```python
from build123d import *

# Parameters (mm, degrees)
BOSS_EXTRUDE2_DEPTH = 331.382
SKETCH3_W           = 66
SKETCH3_H           = 122
CUT_EXTRUDE2_DEPTH  = 128.0000001
SKETCH4_W           = 180
SKETCH4_H           = 60.8
CUT_EXTRUDE3_DEPTH  = 332.3820001
SKETCH5_W           = 260
SKETCH5_H           = 20
CUT_EXTRUDE4_DEPTH  = 332.3820001


with BuildPart() as part:
    # Sketch2 → Boss-Extrude2 (new body)
    with BuildSketch(Plane.XY):
        with BuildLine():
            Line((-127, 127), (127, 127))
            add(Edge.make_bspline(
                [(-127, 127), (0, -127), (127, 127)],
                knots=[0.056028396, 0.056028396, 0.056028396, 0.943971604, 0.943971604, 0.943971604], degree=2))
        make_face()
    extrude(amount=BOSS_EXTRUDE2_DEPTH)

    # Sketch3 → Cut-Extrude2 (cut, through all)
    with BuildSketch(Plane(origin=(0, 127, 0), x_dir=(1, 0, 0), z_dir=(0, 1, 0))):
        with Locations((0, -82.8455)):
            Rectangle(SKETCH3_W, SKETCH3_H)
        with Locations((0, -248.5365)):
            Rectangle(SKETCH3_W, SKETCH3_H)
    extrude(amount=-CUT_EXTRUDE2_DEPTH, mode=Mode.SUBTRACT)

    # Sketch4 → Cut-Extrude3 (cut, through all)
    with BuildSketch(Plane(origin=(0, 0, 0), x_dir=(-1, 0, 0), z_dir=(0, 0, -1))):
        with Locations((0, 30.4)):
            Rectangle(SKETCH4_W, SKETCH4_H)
    extrude(amount=-CUT_EXTRUDE3_DEPTH, mode=Mode.SUBTRACT)

    # Sketch5 → Cut-Extrude4 (cut, through all)
    with BuildSketch(Plane.XY.offset(331.382)):
        with Locations((0, 121.6)):
            Rectangle(SKETCH5_W, SKETCH5_H)
    extrude(amount=-CUT_EXTRUDE4_DEPTH, mode=Mode.SUBTRACT)


solid = part.part
```
Verification items for the finished model (mm, model axes). A direction names the side the tool comes from. Coordinates: 2 decimals unless noted, no trailing zeros. Loops run counter-clockwise (first coordinate to the right, second up) from the corner with the lowest first, then second, coordinate; pieces in that order, holes last. Notation, with made-up numbers: (70.5, -17.75) - (88.5, -17.75) arc R24 cw to (88.5, 19.25) - close; hole circle Ø9 at (32.25, -25.75). An arc over 180 degrees is marked (long way). Return JSON: item names as keys, results as strings.
1. Go/stop test with flat-tipped pins: pin 1 (10 mm diameter, centred on y = 73.5, z = 38.5, fed in from -X); pin 2 (5 mm diameter, centred on y = 66.5, z = 104.5, fed in from -X); pin 3 (10 mm diameter, centred on y = 105, z = 211, fed in from -X). Record where each tip stops, or that it passes through.
Established:
{"pin 1": "stops at x = -99.85", "pin 2": "stops at x = -93.61", "pin 3": "stops at x = -118.19"}
2. Section check A-A, the plane x = -24.5. Record the boundary of the cut face in (y, z), then the cut area to 3 significant figures.
Established:
{"outline": "(60.8, 0) - (111.6, 0) - (111.6, 21.85) - (60.8, 21.85) - close; (60.8, 143.85) - (111.6, 143.85) - (111.6, 187.54) - (60.8, 187.54) - close; (60.8, 309.54) - (111.6, 309.54) - (111.6, 331.38) - (60.8, 331.38) - close", "area": "4,440 mm2"}
3. Thickness scan on L1, parallel to Z at x = 26.5, y = 72; L2, parallel to X at y = 90.5, z = 198; L3, parallel to X at y = 80.5, z = 205.5. Record the ranges inside material, lowest first.
Established:
{"L1": "z = 0 to 21.85, 143.85 to 187.54, 309.54 to 331.38", "L2": "x = -107.21 to -33, 33 to 107.21", "L3": "x = -101.11 to -33, 33 to 101.11"}
4. Tool access check on faces 4 (the flat face through (33, 87, 249)), 5 (the flat face through (2, 87, 0)). Record the directions out of +Z, -Z, +X, -X, +Y, -Y that give a thin tool (end or side, any length) a straight path to the whole face; none if there is none.
Established:
{"face 4": "+Y, -Y", "face 5": "-Z, +X, -X, +Y, -Y"}
5. Mould release check, pull along Z, two halves, no side actions. Record for faces 1 (the flat face through (2, 87, 331.382)), 2 (the flat face through (1, 60.8, 163)), 3 (the flat face through (0, 87, 21.846)): +Z half, -Z half, draft (parallel to the pull), parting line (faces both ways), or undercut.
Established:
{"face 1": "+Z half", "face 2": "draft", "face 3": "undercut"}
6. Section check B-B, the plane y = 93. Count the separate pieces of the cut face and the enclosed holes in it, then the cut area to 3 significant figures.
Established:
{"separate pieces": "1", "enclosed holes": "2", "area": "55,900 mm2"}
